```python
from build123d import *

# Parameters (mm, degrees)
BOSS_EXTRUDE1_DEPTH = 3
CUT_EXTRUDE1_DEPTH  = 4
CUT_EXTRUDE2_DEPTH  = 4


with BuildPart() as part:
    # Sketch1 → Boss-Extrude1 (new body)
    with BuildSketch(Plane.XY):
        Polygon((-10, -13), (-10, -16), (10, -16), (10, -13), (50, -13), (50, 17), (-50, 17), (-50, -13), align=None)
    extrude(amount=BOSS_EXTRUDE1_DEPTH)

    # Sketch2 → Cut-Extrude1 (cut)
    with BuildSketch(Plane.XY.offset(3)):
        Polygon((-50, -13), (1.961524227, 17), (-50, 17), align=None)
    extrude(amount=-CUT_EXTRUDE1_DEPTH, mode=Mode.SUBTRACT)

    # Sketch4 → Cut-Extrude2 (cut)
    with BuildSketch(Plane.XY.offset(3)):
        with BuildLine():
            Line((7.930435314, -0.338457268), (2.930435314, 8.32179677))
            ThreePointArc((2.930435314, 8.32179677), (-0.484628196, 9.236860279), (-1.399691705, 5.82179677))
            Line((-1.399691705, 5.82179677), (3.600308295, -2.838457268))
            ThreePointArc((3.600308295, -2.838457268), (7.015371804, -3.753520778), (7.930435314, -0.338457268))
        make_face()
    extrude(amount=-CUT_EXTRUDE2_DEPTH, mode=Mode.SUBTRACT)


solid = part.part
```
Input: part model. Units: mm. Frame: model coordinates. A direction names the side the tool comes from. Give positions to 0.01 mm unless a question says otherwise; leave off trailing zeros. Loops run counter-clockwise (first coordinate to the right, second up) from the corner with the lowest first, then second, coordinate; pieces in that order, holes last. Notation, with made-up numbers: M 54.25,-35.75 L 67.25,-35.75 A12 ccw 67.25,-15.75 Z; hole C 11.25,58.5 d6. An arc over 180 degrees is marked long. Answer as CSV lines item,"result". Start each with the question number.
1. Section D-D on y = 1. Return loops of the section in (x, z), plus the area to 3 significant figures.
2. Section C-C on x = 17.5. Return loops of the section in (y, z).
3. Pin query (flat end, axial travel): P1, Ø0.9, axis at y = -14.5, z = 1.5, coming from the -X side; P2, Ø1, axis at y = 9.5, z = 1, coming from the -X side; P3, Ø1.5, axis at x = -14, z = 2.5, coming from the +Y side; P4, Ø4, axis at x = 5.5, y = 1.5, coming from the -Z side. Return the tip coordinate at first contact, or that it passes through.
4. Section A-A on z = 1.15. Return loops of the section in (x, y), plus the area to 3 significant figures.
5. Reachability of faces 5 (the face through (-30, -13, 1)), 6 (the face through (0, -16, 1)), 7 (the face through (1.065, 1.552, 1.521)), 8 (the face through (10, -15, 1)) from +Z, -Z, +X, -X, +Y, -Y: full face, straight path, thin tool, end or side. Return the list, or none.
6. Section B-B on y = 7. Return loops of the section in (x, z).
7. Line query: L1, parallel to X at y = 8, z = 0.65; L2, parallel to Y at x = 17, z = 0.85; L3, parallel to X at y = 2, z = 1. Output: solid intervals per line, ascending.
8. Pull-direction query (X, two-part tool) for faces 1 (the face through (-24.38, 1.79, 1.52)), 2 (the face through (-0.44, 9.26, 1.52)), 3 (the face through (6.97, -3.78, 1.52)), 4 (the face through (10, 1, 0)); classes: released by +X, released by -X, zero draft, split by the parting line, or undercut.
Computed values:
1,outline,"M -25.75,0 L 1.38,0 L 1.38,3 L -25.75,3 Z; M 7.16,0 L 50,0 L 50,3 L 7.16,3 Z"
1,area,"210 mm²"
2,outline,"M -13,0 L 17,0 L 17,3 L -13,3 Z"
3,P1,"stops at x = -10"
3,P2,"stops at x = -11.89"
3,P3,"stops at y = 8.22"
3,P4,"stops at z = 0"
4,outline,"M -50,-13 L -10,-13 L -10,-16 L 10,-16 L 10,-13 L 50,-13 L 50,17 L 1.96,17 Z; hole M -1.4,5.82 L 3.6,-2.84 A2.5 ccw 7.93,-0.34 L 2.93,8.32 A2.5 ccw Z"
4,area,"2,210 mm²"
5,face 5,"+Z, -Z, -X, -Y"
5,face 6,"+Z, -Z, +X, -X, -Y"
5,face 7,"+Z, -Z"
5,face 8,"+Z, -Z, +X, -Y"
6,outline,"M -15.36,0 L -1.73,0 L -1.73,3 L -15.36,3 Z; M 3.69,0 L 50,0 L 50,3 L 3.69,3 Z"
7,L1,"x = -13.63 to -1.56, 3.12 to 50"
7,L2,"y = -13 to 17"
7,L3,"x = -24.02 to 0.81, 6.58 to 50"
8,face 1,"released by -X"
8,face 2,"undercut"
8,face 3,"undercut"
8,face 4,"zero draft"
